Drawing for the job (mm, zero at the part's lowest x, y, z). A direction names the side the tool comes from. Round coordinates to 2 decimals unless told otherwise and drop trailing zeros. Write each loop counter-clockwise with the first axis right and the second up, starting at its lowest first coordinate (ties: lowest second). Pieces come first, ordered by that corner, then holes. Notation, with made-up numbers: (-18.75, 43.25) - (16.25, 43.25) arc R19 ccw to (16.25, 54.25) - close; hole circle Ø7 at (32.5, 41.5). An arc over 180 degrees is marked (long way). Answer in a Markdown table with one row per item.
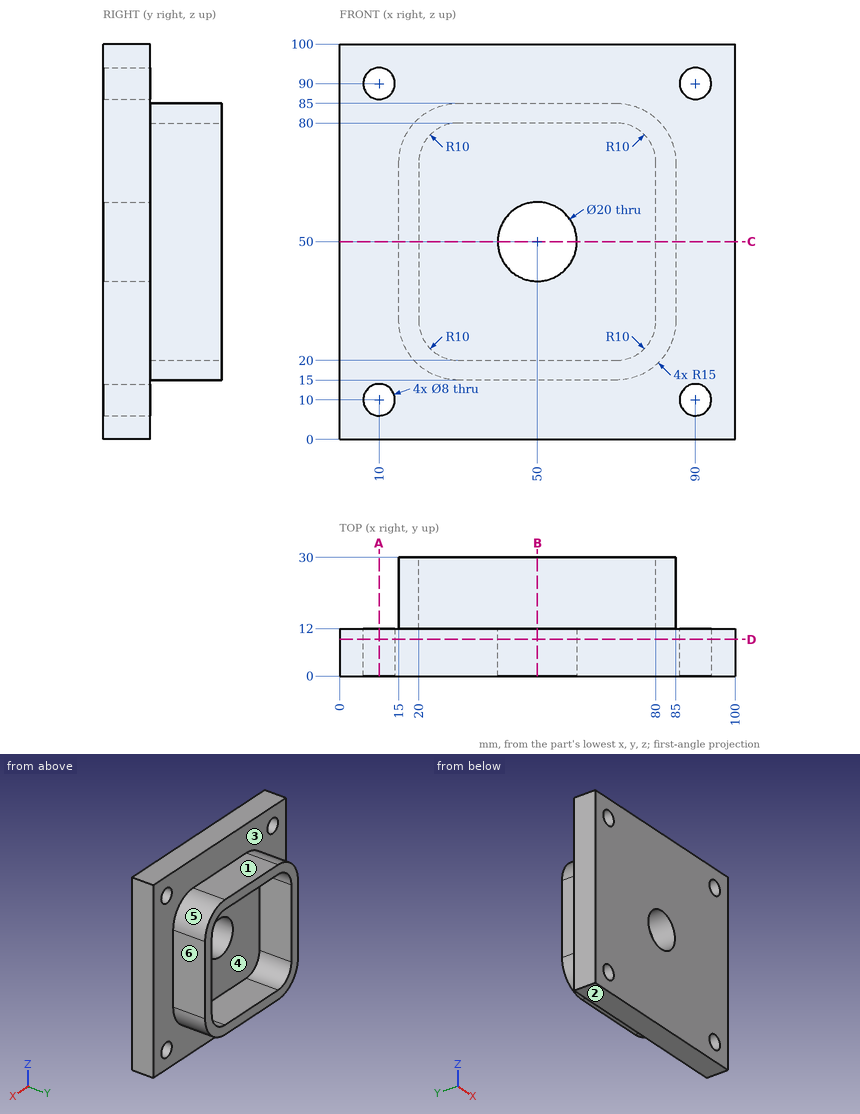
Q1. Saw through at D-D on y = 9.25. List the corners of the cut face in (x, z).
Computed:
| item | result |
|---|---|
| outline | (0, 0) - (100, 0) - (100, 100) - (0, 100) - close; hole circle Ø8 at (10, 10); hole circle Ø8 at (10, 90); hole circle Ø20 at (50, 50); hole circle Ø8 at (90, 10); hole circle Ø8 at (90, 90) |
Q2. Saw through at A-A on x = 10. List the corners of the cut face in (y, z).
Computed:
| item | result |
|---|---|
| outline | (0, 0) - (12, 0) - (12, 6) - (0, 6) - close; (0, 14) - (12, 14) - (12, 86) - (0, 86) - close; (0, 94) - (12, 94) - (12, 100) - (0, 100) - close |
Q3. Flat gauge pins, fed straight in: pin 1 (3 mm diameter, centred on x = 28, y = 16, fed in from -Z); pin 2 (10.5 mm diameter, centred on x = 90, z = 90, fed in from +Y); pin 3 (8 mm diameter, centred on y = 19, z = 46, fed in from +X). Where does each tip first touch, or does it go through?
Computed:
| item | result |
|---|---|
| pin 1 | stops at z = 15.01 |
| pin 2 | stops at y = 12 |
| pin 3 | stops at x = 85 |
Q4. Pull direction Z, two halves, no side cores. Call the marked faces 4, 5 and 6: released by +Z, released by -Z, zero draft, split by the parting line, or undercut.
Computed:
| item | result |
|---|---|
| face 4 | undercut |
| face 5 | released by +Z |
| face 6 | zero draft |
Q5. Drill centre lines: line 1 (Z direction, x = 90, y = 9.5); line 2 (Z direction, x = 34, y = 16.75); line 3 (X direction, y = 7.5, z = 86.5). Where is each one in solid material? Low to high.
Computed:
| item | result |
|---|---|
| line 1 | z = 0 to 6, 14 to 86, 94 to 100 |
| line 2 | z = 15 to 20, 80 to 85 |
| line 3 | x = 0 to 8.06, 11.94 to 88.06, 91.94 to 100 |
Q6. 3-axis set-ups, long thin cutter, end or side, ignore diameter. For the marked faces 1, 2 and 3: which of +Z, -Z, +X, -X, +Y, -Y reach the whole face in a straight line?
Computed:
| item | result |
|---|---|
| face 1 | +Z, +X, -X, +Y |
| face 2 | -Z, +X, -X, +Y, -Y |
| face 3 | +Y |
Q7. Saw through at B-B on x = 50. List the corners of the cut face in (y, z), then the cut area to 3 significant figures.
Computed:
| item | result |
|---|---|
| outline | (0, 0) - (12, 0) - (12, 15) - (30, 15) - (30, 20) - (12, 20) - (12, 40) - (0, 40) - close; (0, 60) - (12, 60) - (12, 80) - (30, 80) - (30, 85) - (12, 85) - (12, 100) - (0, 100) - close |
| area | 1,140 mm2 |
Q8. Saw through at C-C on z = 50. List the corners of the cut face in (x, y).
Computed:
| item | result |
|---|---|
| outline | (0, 0) - (40, 0) - (40, 12) - (20, 12) - (20, 30) - (15, 30) - (15, 12) - (0, 12) - close; (60, 0) - (100, 0) - (100, 12) - (85, 12) - (85, 30) - (80, 30) - (80, 12) - (60, 12) - close |
